Answer from the drawing. Dimensions are ordinates in mm from the lowest x, y and z of the part. Coordinates: 2 decimals unless noted, no trailing zeros. Write each loop counter-clockwise with the first axis right and the second up, starting at its lowest first coordinate (ties: lowest second). Pieces come first, ordered by that corner, then holes. Notation, with made-up numbers: (-6, 53.25) - (12, 53.25) arc R22 cw to (12, 67.25) - close; hole circle Ø3 at (16.25, -27). An arc over 180 degrees is marked (long way). Answer as a JSON object with one key per item and string values. Group by question number.
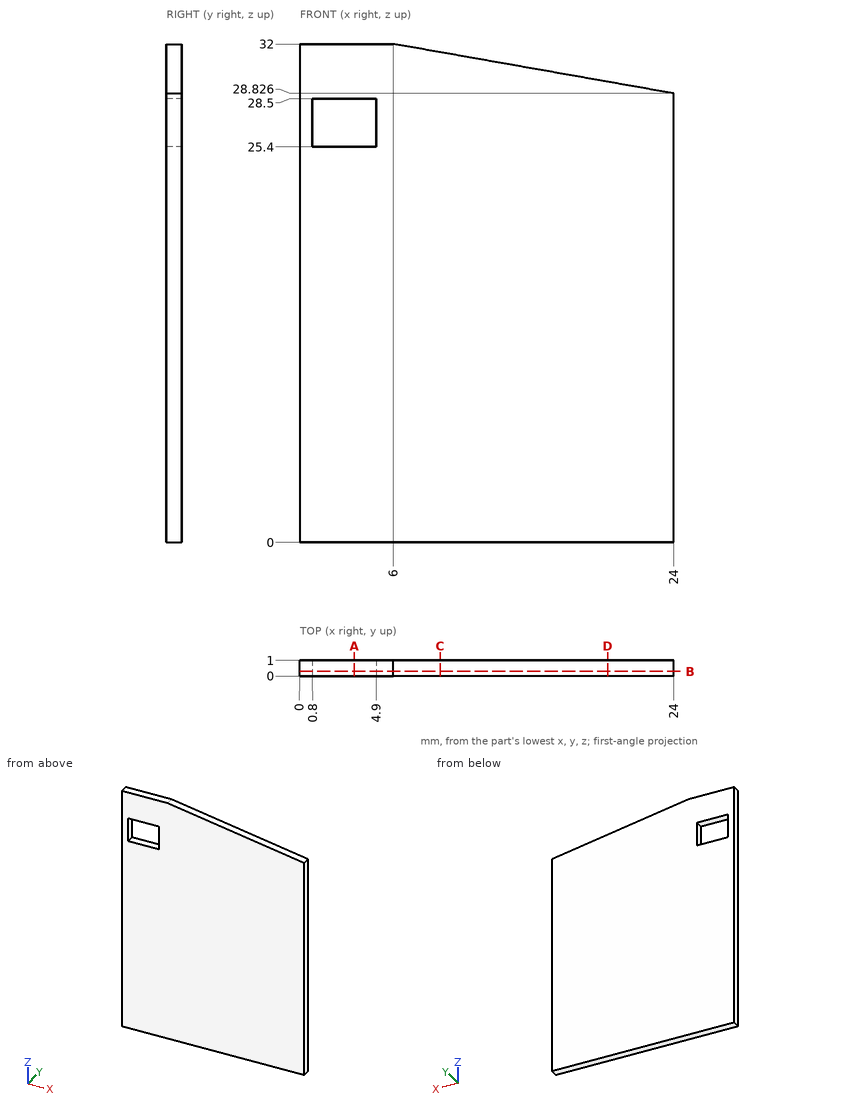
Q1. Consider L1, parallel to Z at x = 4.25, y = 0.1; L2, parallel to Z at x = 15.5, y = 0.25 (3 decimals); L3, parallel to Z at x = 17.5, y = 0.8. Determine where each line is inside the solid, lowest interval first. Write a range as from..to.
Q2. Section B-B on y = 0.3 is taken. Determine the outline of the cut face in (x, z), plus the area to 3 significant figures.
Q3. Section D-D on x = 19.75 is taken. Determine the outline of the cut face in (y, z), plus the area to 3 significant figures.
Q4. A flat-ended cylindrical pin translates along its axis: pin 1 Ø2 at (x, z) = (3.5, 22.5) entering from -Y. Find the tip coordinate at first contact, or state that the pin passes through.
Q5. Section A-A on x = 3.5 is taken. Determine the outline of the cut face in (y, z).
Q6. Section C-C on x = 9 is taken. Determine the outline of the cut face in (y, z).
Numbers:
{
 "1": {"L1": "z = 0..25.4, 28.5..32", "L2": "z = 0..30.325", "L3": "z = 0..29.97"},
 "2": {"outline": "(0, 0) - (24, 0) - (24, 28.83) - (6, 32) - (0, 32) - close; hole (0.8, 25.4) - (4.9, 25.4) - (4.9, 28.5) - (0.8, 28.5) - close", "area": "727 mm²"},
 "3": {"outline": "(0, 0) - (1, 0) - (1, 29.58) - (0, 29.58) - close", "area": "29.6 mm²"},
 "4": {"pin 1": "stops at y = 0"},
 "5": {"outline": "(0, 0) - (1, 0) - (1, 25.4) - (0, 25.4) - close; (0, 28.5) - (1, 28.5) - (1, 32) - (0, 32) - close"},
 "6": {"outline": "(0, 0) - (1, 0) - (1, 31.47) - (0, 31.47) - close"}
}
